Could you check a few things on this model? Use its own coordinates, in mm. A direction names the side the tool comes from. Round coordinates to 2 decimals unless told otherwise and drop trailing zeros. Loops run counter-clockwise (first coordinate to the right, second up) from the corner with the lowest first, then second, coordinate; pieces in that order, holes last. Notation, with made-up numbers: (79.25, -10.5) - (116.25, -10.5) arc R20 ccw to (116.25, 14.5) - close; hole circle Ø3 at (6, 18). An arc over 180 degrees is marked (long way). Use one line per item in the form item = value.
```python
from build123d import *

# Parameters (mm, degrees)
SKETCH1_W           = 19.4
SKETCH1_H           = 1.4
BOSS_EXTRUDE1_DEPTH = 35
BOSS_EXTRUDE2_DEPTH = 1.7


with BuildPart() as part:
    # Sketch1 → Boss-Extrude1 (new body)
    with BuildSketch(Plane.XY):
        with Locations((9.7, 0.7)):
            Rectangle(SKETCH1_W, SKETCH1_H)
    extrude(amount=BOSS_EXTRUDE1_DEPTH)

    # Sketch3 → Boss-Extrude2 (add)
    with BuildSketch(Plane(origin=(0, 1.4, 0), x_dir=(1, 0, 0), z_dir=(0, 1, 0))):
        with BuildLine():
            Line((3.679202711, -35), (3.679202711, -35.789714785))
            ThreePointArc((3.679202711, -35.789714785), (3.719569751, -35.986533337), (3.83415288, -36.151571959))
            ThreePointArc((3.83415288, -36.151571959), (9.7, -38.5), (15.56584712, -36.151571959))
            ThreePointArc((15.56584712, -36.151571959), (15.680430249, -35.986533337), (15.720797289, -35.789714785))
            Line((15.720797289, -35.789714785), (15.720797289, -35))
            Line((15.720797289, -35), (14.720797289, -35))
            Line((14.720797289, -35), (14.720797289, -35.741493674))
            ThreePointArc((14.720797289, -35.741493674), (14.663106522, -35.974651436), (14.50334712, -36.154004999))
            ThreePointArc((14.50334712, -36.154004999), (9.7, -37.641312474), (4.89665288, -36.154004999))
            ThreePointArc((4.89665288, -36.154004999), (4.736893478, -35.974651436), (4.679202711, -35.741493674))
            Line((4.679202711, -35.741493674), (4.679202711, -35))
            Line((4.679202711, -35), (3.679202711, -35))
        make_face()
    extrude(amount=-BOSS_EXTRUDE2_DEPTH)


solid = part.part
```
1. If we section it at D-D, the plane x = 2.5: Write out the boundary of the cut face in (y, z), plus the area to 3 significant figures.
Solution:
outline = (0, 0) - (1.4, 0) - (1.4, 35) - (0, 35) - close
area = 49.0 mm^2
2. If we section it at A-A, the plane y = 1: Write out the boundary of the cut face in (x, z), plus the area to 3 significant figures.
Solution:
outline = (0, 0) - (19.4, 0) - (19.4, 35) - (15.72, 35) - (15.72, 35.79) arc R0.5 ccw to (15.57, 36.15) arc R8.5 ccw to (3.83, 36.15) arc R0.5 ccw to (3.68, 35.79) - (3.68, 35) - (0, 35) - close; hole (4.68, 35) - (14.72, 35) - (14.72, 35.74) arc R0.5 ccw to (14.5, 36.15) arc R8.5 ccw to (4.9, 36.15) arc R0.5 ccw to (4.68, 35.74) - close
area = 691 mm^2
3. If we section it at B-B, the plane x = 12.25: Write out the boundary of the cut face in (y, z).
Solution:
outline = (-0.3, 37.25) - (1.4, 37.25) - (1.4, 38.11) - (-0.3, 38.11) - close; (0, 0) - (1.4, 0) - (1.4, 35) - (0, 35) - close
4. For P1, Ø0.7, axis at x = 17, y = 1, coming from the +Z side; P2, Ø6, axis at x = 13.5, z = 19.5, coming from the -Y side, each with a flat end and sliding along its axis, tell me the tip position at first contact or that it passes through.
Solution:
P1 = 35
P2 = 0
5. If we section it at C-C, the plane z = 7.5: Write out the boundary of the cut face in (x, y).
Solution:
outline = (0, 0) - (19.4, 0) - (19.4, 1.4) - (0, 1.4) - close
6. We'd pull the mould along Z, two halves only. Please class faces 6 (the face through (0, 1, 17)), 7 (the face through (9.6, 0.6, 38.5)), 8 (the face through (10, 1, 35)): +Z half, -Z half, draft (parallel to the pull), parting line (faces both ways), or undercut.
Solution:
face_6 = draft
face_7 = +Z half
face_8 = undercut
7. Please list where these lines run through material, in increasing order: line 1 along Y through (x, z) = (5, 27.5); line 2 along X through (y, z) = (0.2, 35.5); line 3 along Z through (x, y) = (13, 0.3).
Solution:
line_1 = 0 to 1.4
line_2 = 3.68 to 4.68, 14.72 to 15.72
line_3 = 0 to 35, 36.97 to 37.83
8. On a 3-axis mill with a long thin cutter (end or side, diameter ignored), from which of +Z, -Z, +X, -X, +Y, -Y can I reach the whole of each face in a straight line? I mean faces 1 (the face through (10, 0, 17)), 2 (the face through (9.77, 0.56, 37.64)), 3 (the face through (18, 1, 35)), 4 (the face through (19.4, 1, 17)), 5 (the face through (2, 1, 35)). Say none if no direction works.
Solution:
face_1 = -Z, +X, -X, -Y
face_2 = +Y, -Y
face_3 = +Z, +X, +Y, -Y
face_4 = +Z, -Z, +X, +Y, -Y
face_5 = +Z, -X, +Y, -Y
